CAD build for the part. Positions are in the model's coordinates, mm. A direction names the side the tool comes from. Round coordinates to 2 decimals unless told otherwise and drop trailing zeros. Order: outer loops, then holes, each group sorted by start corner. A loop starts at its lowest first (then second) coordinate and runs counter-clockwise, first axis right, second up. Notation, with made-up numbers: M 72,41.25 L 85,41.25 A9 ccw 85,53.25 Z; hole C -11,41 d8. An arc over 180 degrees is marked long. Answer as a JSON object with one key per item and string values.
Autodesk Inventor part; units mm, degrees
ref_plane "Work Plane4" through (27.5, 27.5, 4) normal (0.7071, -0.7071, 0) x (0, 0, 1)
ref_plane "YZ Plane" through (0, 0, 0) normal (1, 0, 0) x (0, 1, 0)
ref_plane "XZ Plane" through (0, 0, 0) normal (0, 1, 0) x (-1, 0, 0)
sketch "Sketch1" plane through (0, 0, 0) normal (0, 0, 1) x (1, 0, 0)
  line L0 (0, 0) -> (44, 0)
  line L1 (44, 0) -> (44, 44)
  line L2 (44, 44) -> (0, 44)
  line L3 (0, 44) -> (0, 0)
  line L4 (0, 0) -> (0.5, 0)
  line L5 (0.5, 0) -> (0.5, 0.5)
  line L6 (0.5, 0.5) -> (43.5, 0.5)
  line L7 (43.5, 0.5) -> (43.5, 43.5)
  line L8 (43.5, 43.5) -> (0.5, 43.5)
  line L9 (0.5, 43.5) -> (0.5, 0.5)
  dimension "d0" = 44
  dimension "d1" = 44
  dimension "d103" = 0.5
  dimension "d104" = 0.5
  dimension "d105" = 43
  dimension "d106" = 43
extrude "Extrusion1" add sketch "Sketch1" along normal blind 4 contours L9 L8 L7 L6
chamfer "Chamfer1" distance 4 angle 45 4 edges at (43.5, 22, 4) (22, 0.5, 4) (0.5, 22, 4) (22, 43.5, 4)
sketch "Sketch2" plane through (0, 0, 4) normal (0, 0, 1) x (1, 0, 0)
  line L0 (4, 4) -> (40, 40)
  line L1 (22, 16.5) -> (16.5, 16.5)
  line L2 (16.5, 16.5) -> (16.5, 27.5)
  line L3 (16.5, 27.5) -> (27.5, 27.5)
  line L4 (27.5, 27.5) -> (27.5, 16.5)
  line L5 (27.5, 16.5) -> (22, 16.5)
  line L6 (27.5, 27.5) -> (27.5, 25.5)
  arc A0 (18.5, 27.5) -> (16.5, 25.5) centre (18.5, 25.5) ccw
  line L7 (18.5, 25.5) -> (18.5, 18.5)
  line L8 (18.5, 18.5) -> (25.5, 18.5)
  line L9 (25.5, 18.5) -> (25.5, 25.5)
  arc A1 (16.5, 18.5) -> (18.5, 16.5) centre (18.5, 18.5) ccw
  arc A2 (25.5, 16.5) -> (27.5, 18.5) centre (25.5, 18.5) ccw
  arc A3 (27.5, 25.5) -> (25.5, 27.5) centre (25.5, 25.5) ccw
  line L10 (27.5, 18.5) -> (25.5, 16.5)
  line L11 (18.5, 16.5) -> (16.5, 18.5)
  line L12 (16.5, 25.5) -> (18.5, 27.5)
  line L13 (25.5, 27.5) -> (27.5, 25.5)
  point P0 (0, 0)
  dimension "d86" = 2
extrude "Extrusion2" cut sketch "Sketch2" against normal blind 3 contours L0 L11 L2 L12 L3 L13 | L8 L9 L0 L13 L4 L10 L5 L1 L11 | L0 L9 L8
ref_plane "Work Plane4" through (27.5, 27.5, 4) normal (0.7071, -0.7071, 0) x (0, 0, 1)
sketch "Sketch15" plane through (0, 0, 4) normal (0, 0, 1) x (1, 0, 0)
  line L0 (18.5, 16.5) -> (16.5, 18.5)
  line L1 (16.5, 18.5) -> (16.5, 25.5)
  line L2 (16.5, 25.5) -> (18.5, 27.5)
  line L3 (18.5, 27.5) -> (25.5, 27.5)
  line L4 (25.5, 27.5) -> (27.5, 25.5)
  line L5 (27.5, 25.5) -> (27.5, 18.5)
  line L6 (27.5, 18.5) -> (25.5, 16.5)
  line L7 (25.5, 16.5) -> (18.5, 16.5)
  line L8 (16.5, 18.5) -> (16.5, 25.5)
  line L9 (15, 22.9038) -> (15, 29)
  line L10 (15, 29) -> (29, 29)
  line L11 (29, 29) -> (29, 15)
  line L12 (29, 15) -> (15, 15)
  line L13 (15, 15) -> (15, 29)
  line L14 (16.5, 18.5) -> (16.5, 16.5)
  line L15 (16.5, 16.5) -> (18.5, 16.5)
  line L16 (25.5, 16.5) -> (27.5, 16.5)
  line L17 (27.5, 16.5) -> (27.5, 18.5)
  line L18 (27.5, 25.5) -> (27.5, 27.5)
  line L19 (25.5, 27.5) -> (27.5, 25.5)
  line L20 (27.5, 27.5) -> (25.5, 27.5)
  line L21 (18.5, 27.5) -> (16.5, 27.5)
  line L22 (16.5, 27.5) -> (16.5, 25.5)
  point P0 (0, 0)
extrude "Extrusion7" add sketch "Sketch15" along normal blind 2.5
chamfer "Chamfer6" distance 1.5 angle 45 4 edges at (22, 16.5, 6.5) (16.5, 22, 6.5) (27.5, 22, 6.5) (22, 27.5, 6.5)
sketch "Sketch16" plane through (0, 0, 4) normal (0, 0, 1) x (1, 0, 0)
  line L0 (16.5, 18.5) -> (16.5, 16.5)
  line L1 (16.5, 16.5) -> (18.5, 16.5)
  line L2 (18.5, 16.5) -> (16.5, 18.5)
  line L3 (27.5, 16.5) -> (27.5, 18.5)
  line L4 (27.5, 18.5) -> (25.5, 16.5)
  line L5 (25.5, 16.5) -> (27.5, 16.5)
  line L6 (25.5, 27.5) -> (27.5, 25.5)
  line L7 (27.5, 27.5) -> (25.5, 27.5)
  line L8 (25.5, 27.5) -> (27.5, 25.5)
  line L9 (27.5, 25.5) -> (27.5, 27.5)
  line L10 (18.5, 27.5) -> (16.5, 27.5)
  line L11 (16.5, 27.5) -> (16.5, 25.5)
  line L12 (16.5, 25.5) -> (18.5, 27.5)
  point P0 (0, 0)
extrude "Extrusion8" add sketch "Sketch16" along normal blind 1
ref_plane "Work Plane6" through (22, 18.5, 1) normal (-1, 0, 0) x (0, 0, 1)
ref_plane "Work Plane7" through (18.5, 22, 1) normal (0, 1, 0) x (1, 0, 0)
sketch "Sketch17" plane through (18.5, 22, 1) normal (0, 1, 0) x (1, 0, 0)
  line L0 (7, -4) -> (7, 0)
  line L1 (7, 0) -> (0, 0)
  line L2 (0, -4) -> (0, 0)
  line L3 (7, -4) -> (0, -4)
  line L4 (3.5, 0) -> (2.25, 0)
  line L5 (2.25, 0) -> (2.25, -2.5)
  line L6 (2.25, -2.5) -> (4.75, -2.5)
  line L7 (4.75, -2.5) -> (4.75, 0)
  point P0 (-18.5, 1)
  dimension "d109" = 1.25
  dimension "d110" = 2.5
  dimension "d111" = 2.5
sketch "Sketch18" plane through (22, 18.5, 1) normal (-1, 0, 0) x (0, 0, 1)
  line L0 (4, 7) -> (0, 7)
  line L1 (0, 7) -> (0, 0)
  line L2 (4, 0) -> (0, 0)
  line L3 (4, 7) -> (4, 0)
  line L4 (0, 3.5) -> (1.25, 3.5)
  line L5 (1.25, 3.5) -> (1.25, -6.5)
  line L6 (1.25, -6.5) -> (6.9224, -12.1724)
  line L7 (1.25, 3.5) -> (1.25, 4.137)
  line L8 (1.25, 4.137) -> (1.25, 14.137)
  line L9 (1.25, 14.137) -> (10.5582, 23.4452)
  point P0 (-1, -18.5)
  dimension "d113" = 10
  dimension "d114" = 135
sweep "Sweep4" cut profiles "Sketch17" path "Sketch18" path curves L5 L6 contours L7 L6 L5 L1
sweep "Sweep5" cut profiles "Sketch17" path "Sketch18" path curves L7 L8 L9 contours L7 L6 L5 L1
ref_plane "Work Plane8" through (18.5, 24, 1) normal (0, 1, 0) x (1, 0, 0)
sketch "Sketch19" plane through (22, 18.5, 1) normal (-1, 0, 0) x (0, 0, 1)
  line L0 (-2.3, 5.5) -> (6.8, 5.5)
  line L1 (4, 7) -> (0, 7)
  line L2 (0, 7) -> (0, 0)
  line L3 (4, 0) -> (0, 0)
  line L4 (4, 7) -> (4, 0)
  line L5 (4, 0) -> (4, 7)
  line L6 (4, 5.5) -> (4, 4.25)
  line L7 (4, 4.25) -> (1.5, 4.25)
  line L8 (1.5, 4.25) -> (1.5, 6.75)
  line L9 (1.5, 6.75) -> (4, 6.75)
  line L10 (4, 6.75) -> (4, 4.25)
  point P0 (-1, -18.5)
  dimension "d127" = 1.25
  dimension "d128" = 2.5
  dimension "d129" = 2.5
sketch "Sketch20" plane through (18.5, 24, 1) normal (0, 1, 0) x (1, 0, 0)
  line L0 (3.5, 2.3) -> (3.5, -6.8)
  line L1 (3.5, -4) -> (3.5, -2.75)
  line L2 (3.5, -2.75) -> (-6.5, -2.75)
  line L3 (-6.5, -2.75) -> (-11.0554, -7.3054)
  line L4 (3.5, -2.75) -> (13.5, -2.75)
  line L5 (13.5, -2.75) -> (17.1075, -6.3575)
  point P0 (-18.5, 1)
  point P1 (3.5, -4)
  dimension "d130" = 1.25
  dimension "d131" = 10
  dimension "d132" = 135
  dimension "d134" = 10
sweep "Sweep6" cut profiles "Sketch19" path "Sketch20" path curves L5 L4 L2 L3 contours L8 L9 L4 L0 | L0 L4 L7 L8
properties part number "clear-square-reed-2"
Item 1: Two-plate mould, pull along X, no slides. Class faces 5 (the flat face through (27.5, 21, 3)), 6 (the flat face through (41.5, 22.3, 2)), 7 (the flat face through (22, 29, 5)), 8 (the flat face through (13, 22.75, 3)): released by +X, released by -X, zero draft, split by the parting line, or undercut.
Worked answers:
{"face 5": "undercut", "face 6": "released by +X", "face 7": "zero draft", "face 8": "undercut"}
Item 2: Wall check: line 1 along X through (y, z) = (22, 2); line 2 along Y through (x, z) = (26, 2.75); line 3 along Y through (x, z) = (19, 5.25). Give the ranges that are in metal, low to high. Write a range as [from, to].
Worked answers:
{"line 1": "x = [2.5, 16.5], [27.5, 41.5]", "line 2": "y = [3.25, 17], [27, 40.75]", "line 3": "y = [15, 16.25], [27.75, 29]"}
Item 3: Saw through at C-C on z = 5.75. List the corners of the cut face in (x, y).
Worked answers:
{"outline": "M 15,15 L 29,15 L 29,29 L 15,29 Z; hole M 15.75,15.75 L 28.25,15.75 L 28.25,28.25 L 15.75,28.25 Z"}
Item 4: 3-axis set-ups, long thin cutter, end or side, ignore diameter. For faces 1 (the flat face through (23.25, 13, 3)), 2 (the flat face through (22, 15, 5)), 3 (the flat face through (29, 22, 5)), 4 (the flat face through (22.1, 28.2, 5.7)): which of +Z, -Z, +X, -X, +Y, -Y reach the whole face in a straight line?
Worked answers:
{"face 1": "none", "face 2": "+Z, +X, -X, -Y", "face 3": "+Z, +X, +Y, -Y", "face 4": "+Z"}
Item 5: Drop flat-ended pins along their axis: pin 1 Ø1.2 at (x, z) = (14.5, 3) entering from -Y; pin 2 Ø1.6 at (x, y) = (26.5, 26.5) entering from +Z; pin 3 Ø3 at (x, y) = (38, 10) entering from +Z. Give the stop position or say it passes through.
Worked answers:
{"pin 1": "stops at y = 2.9", "pin 2": "stops at z = 5", "pin 3": "stops at z = 4"}
